Source: CAD feature listing. Evaluate the final solid. Frame: model axes, mm. Face numbers are marked on the shaded views. A direction names the side the tool comes from. Give positions to 0.01 mm unless a question says otherwise; leave off trailing zeros. Order: outer loops, then holes, each group sorted by start corner. A loop starts at its lowest first (then second) coordinate and runs counter-clockwise, first axis right, second up. Notation, with made-up numbers: (8.25, 22.5) -> (62.25, 22.5) arc R22 cw to (62.25, 46.5) -> close; hole circle Ø2 at (7, 5.5). An arc over 180 degrees is marked (long way). Answer in a Markdown table with one row per item.
```python
from build123d import *

# Parameters (mm, degrees)
SKETCH1_R                      = 14.6812
SKETCH1_R_2                    = 11.5062
BEARING_INSERT_EXTRUDE_DEPTH   = 4.7625
APEX_SLOT_INSERT_EXTRUDE_DEPTH = 3.175
FILLET1_R                      = 5.08
FILLET2_R                      = 2.8575


with BuildPart() as part:
    # Sketch1 → Bearing_Insert_Extrude (new, symmetric)
    with BuildSketch(Plane(origin=(0, 0, 0), x_dir=(1, 0, 0), z_dir=(0, 1, 0))):
        with Locations(Location((0, 0, 0), (0, 0, 90))):
            Circle(SKETCH1_R)
        with Locations(Location((0, 0, 0), (0, 0, 90))):
            Circle(SKETCH1_R_2, mode=Mode.SUBTRACT)
    extrude(amount=BEARING_INSERT_EXTRUDE_DEPTH, both=True)

    # Sketch1<4> → Apex_Slot_Insert_Extrude (add, symmetric)
    with BuildSketch(Plane(origin=(0, 0, 0), x_dir=(1, 0, 0), z_dir=(0, 1, 0))):
        with BuildLine():
            Line((-10.414, -10.348248037), (-10.414, -55.88))
            Line((-10.414, -55.88), (10.414, -55.88))
            Line((10.414, -55.88), (10.414, -27.365061948))
            Line((10.414, -27.365061948), (29.371655227, -48.665507962))
            Line((29.371655227, -48.665507962), (44.930015858, -34.818378351))
            Line((44.930015858, -34.818378351), (14.659031085, -0.806499284))
            ThreePointArc((14.659031085, -0.806499284), (5.221715671, -13.721199616), (-10.414, -10.348248037))
        make_face()
        with BuildLine():
            ThreePointArc((6.096, -45.0215), (0, -51.1175), (-6.096, -45.0215))
            Line((-6.096, -45.0215), (-6.096, -27.2415))
            ThreePointArc((-6.096, -27.2415), (0, -21.1455), (6.096, -27.2415))
            Line((6.096, -27.2415), (6.096, -45.0215))
        make_face(mode=Mode.SUBTRACT)
        with BuildLine():
            ThreePointArc((34.485419253, -29.577906234), (33.98457115, -38.184391183), (25.378086201, -37.68354308))
            Line((25.378086201, -37.68354308), (13.557365801, -24.402015712))
            ThreePointArc((13.557365801, -24.402015712), (14.058213904, -15.795530763), (22.664698853, -16.296378866))
            Line((22.664698853, -16.296378866), (34.485419253, -29.577906234))
        make_face(mode=Mode.SUBTRACT)
    extrude(amount=APEX_SLOT_INSERT_EXTRUDE_DEPTH, both=True)

    # Fillet1
    fillet1_edges = [part.edges().sort_by_distance(p)[0] for p in [
        (14.659031085, 0, 0.806499284),
        (-10.414, 0, 10.348248037),
    ]]
    fillet(fillet1_edges, radius=FILLET1_R)

    # Fillet2
    fillet2_edges = [part.edges().sort_by_distance(p)[0] for p in [
        (-10.414, 0, 55.88),
        (10.414, 0, 55.88),
        (10.414, 0, 27.365061948),
        (29.371655227, 0, 48.665507962),
        (44.930015858, 0, 34.818378351),
    ]]
    fillet(fillet2_edges, radius=FILLET2_R)


solid = part.part
```
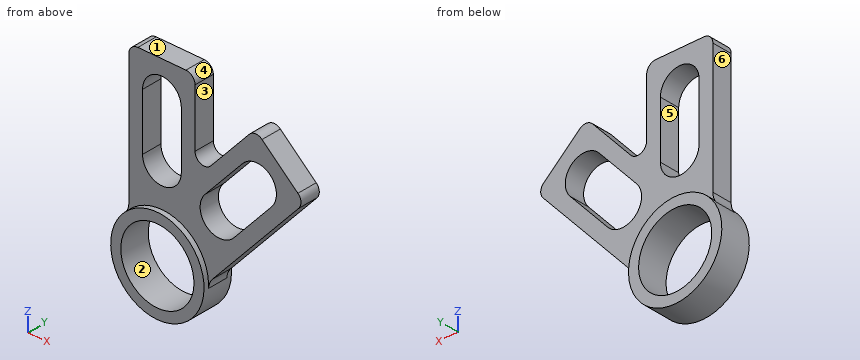
(1) Section query D-D (z = 18.5). Return the cut outline in (x, y) (3 decimals).
A:
| item | result |
|---|---|
| outline | (-10.414, -3.175) -> (12.302, -3.175) -> (12.302, 3.175) -> (-10.414, 3.175) -> close; (24.626, -3.175) -> (30.406, -3.175) -> (30.406, 3.175) -> (24.626, 3.175) -> close |
(2) Section query A-A (x = 0). Return the cut outline in (y, z) (1 decimal).
A:
| item | result |
|---|---|
| outline | (-4.8, -14.7) -> (4.8, -14.7) -> (4.8, -11.5) -> (-4.8, -11.5) -> close; (-4.8, 11.5) -> (4.8, 11.5) -> (4.8, 14.7) -> (3.2, 14.7) -> (3.2, 21.1) -> (-3.2, 21.1) -> (-3.2, 14.7) -> (-4.8, 14.7) -> close; (-3.2, 51.1) -> (3.2, 51.1) -> (3.2, 55.9) -> (-3.2, 55.9) -> close |
(3) Pull-direction query (Z, two-part tool) for the marked faces 1, 2 and 3; classes: +Z half, -Z half, draft (parallel to the pull), parting line (faces both ways), or undercut.
A:
| item | result |
|---|---|
| face 1 | +Z half |
| face 2 | undercut |
| face 3 | draft |
(4) First-contact query: pin 1 Ø4 at (x, y) = (18.5, 2) entering from +Z; pin 2 Ø1 at (y, z) = (-0.5, 29) entering from -X; pin 3 Ø3 at (y, z) = (-1.5, 38.5) entering from +X. Flat tips, straight axial feed; report the tip coordinate or a pass-through.
A:
| item | result |
|---|---|
| pin 1 | stops at z = 38.7 |
| pin 2 | stops at x = -10.41 |
| pin 3 | stops at x = 42.48 |
(5) Section query C-C (y = -0.25). Return the cut outline in (x, z) (1 decimal), plus the area to 3 significant figures.
A:
| item | result |
|---|---|
| outline | (-11.5, 9.1) arc R14.7 ccw (long way) to (14.7, -0.8) arc R5.1 cw to (15.9, 2.2) -> (43, 32.7) arc R2.9 ccw to (42.8, 36.7) -> (31.5, 46.8) arc R2.9 ccw to (27.5, 46.5) -> (15.4, 33) arc R2.9 cw to (10.4, 34.9) -> (10.4, 53) arc R2.9 ccw to (7.6, 55.9) -> (-7.6, 55.9) arc R2.9 ccw to (-10.4, 53) -> (-10.4, 12.3) arc R5.1 cw to start; hole circle Ø23 at (0, 0); hole (-6.1, 27.2) arc R6.1 ccw to (6.1, 27.2) -> (6.1, 45) arc R6.1 ccw to (-6.1, 45) -> close; hole (13.6, 24.4) arc R6.1 ccw to (22.7, 16.3) -> (34.5, 29.6) arc R6.1 ccw to (25.4, 37.7) -> close |
| area | 1,290 mm^2 |
(6) Access query for the marked faces 4, 5 and 6. Directions: +Z, -Z, +X, -X, +Y, -Y. A direction counts if a zero-diameter tool reaches every point of the face in a straight line with its end or side. Return the directions, or none.
A:
| item | result |
|---|---|
| face 4 | +Z, +X, +Y, -Y |
| face 5 | +Y, -Y |
| face 6 | +Z, -X, +Y, -Y |
(7) Ray query, probe 1 along X at (y, z) = (3, 43.5); probe 2 along X at (y, z) = (2.5, 24); probe 3 along X at (y, z) = (-0.5, 0). Return the intervals inside material, ascending.
A:
| item | result |
|---|---|
| probe 1 | x = -10.41 to -6.1, 6.1 to 10.41, 24.77 to 35.18 |
| probe 2 | x = -10.41 to -5.16, 5.16 to 13.23, 29.52 to 35.3 |
| probe 3 | x = -14.68 to -11.51, 11.51 to 14.78 |
(8) Section query B-B (z = 42). Return the cut outline in (x, y) (3 decimals).
A:
| item | result |
|---|---|
| outline | (-10.414, -3.175) -> (-6.096, -3.175) -> (-6.096, 3.175) -> (-10.414, 3.175) -> close; (6.096, -3.175) -> (10.414, -3.175) -> (10.414, 3.175) -> (6.096, 3.175) -> close; (23.439, -3.175) -> (36.861, -3.175) -> (36.861, 3.175) -> (23.439, 3.175) -> close |
